```python
from build123d import *

# Parameters (mm, degrees)
F1_DEPTH = 101.6
F2_W     = 62.789462
F2_H     = 290.428608
F3_DEPTH = 76.2
F4_R     = 26.772602
F5_DEPTH = 101.6
F6_R     = 12.094446
F6_R_2   = 13.485849
F7_DEPTH = 101.6


with BuildPart() as f1:
    # F0 (on Front) → F1 (new body)
    with BuildSketch(Plane.XZ):
        with BuildLine():
            Line((27.304832, -72.607152), (27.304832, 72.607152))
            ThreePointArc((27.304832, 72.607152), (0, 99.911984), (-27.304832, 72.607152))
            Line((-27.304832, 72.607152), (-27.304832, -72.607152))
            ThreePointArc((-27.304832, -72.607152), (0, -99.911984), (27.304832, -72.607152))
        make_face()
    extrude(amount=-F1_DEPTH)

    # F2 (on face) → F3 (cut)
    with BuildSketch(Plane.YZ.offset(27.304832)):
        with Locations((50.8, 72.607152)):
            Rectangle(F2_W, F2_H)
    extrude(amount=-F3_DEPTH, mode=Mode.SUBTRACT)

    # F4 (on Front) → F5 (join)
    with BuildSketch(Plane.XZ):
        with Locations((0, -72.568707)):
            Circle(F4_R)
    extrude(amount=-F5_DEPTH)

    # F6 (on face) → F7 (cut)
    with BuildSketch(Plane.XZ):
        with Locations((0, 75.886309)):
            Circle(F6_R)
        with Locations((0, -72.607152)):
            Circle(F6_R_2)
    extrude(amount=-F7_DEPTH, mode=Mode.SUBTRACT)


solid = f1.part
```
CAD build for the part. Positions are in the model's coordinates, mm. Coordinates: 2 decimals unless noted, no trailing zeros. Write each loop counter-clockwise with the first axis right and the second up, starting at its lowest first coordinate (ties: lowest second). Pieces come first, ordered by that corner, then holes.
(1) Flat gauge pins, fed straight in: pin 1 (1.5 mm diameter, centred on y = 79.5, z = -56, fed in from -X); pin 2 (8 mm diameter, centred on y = 36, z = -46.5, fed in from -X); pin 3 (2 mm diameter, centred on x = 2.5, y = 74, fed in from +Z). Where does each tip first touch, or does it go through?
(2) Cut at B-B, the plane z = 26. List the corners of the cut face in (x, y), and give its area (3 significant figures).
(3) Cut at D-D, the plane y = 13. List the corners of the cut face in (x, z).
(4) Cut at A-A, the plane x = 0. List the corners of the cut face in (y, z).
(5) Two-plate mould, pull along Y, no slides. Class faces 1 (the face through (0, 0, 1)), 2 (the face through (0, 82.195, 12)), 3 (the face through (-0.6, 50.089, -99.905)): +Y half, -Y half, draft (parallel to the pull), parting line (faces both ways), or undercut.
(6) Cut at C-C, the plane y = 62.5. List the corners of the cut face in (x, z), and give its area (3 significant figures).
(7) Drill centre lines: probe 1 along Z at (x, y) = (0, 93); probe 2 along Z at (x, y) = (0, 47); probe 3 along Y at (x, z) = (-18, 41). Where is each one in solid material? Low to high.
Geometry says:
1. pin 1: stops at x = -21.6
1. pin 2: stops at x = -15.16
1. pin 3: stops at z = -45.84
2. outline: (-27.3, 0) - (27.3, 0) - (27.3, 19.41) - (-27.3, 19.41) - close; (-27.3, 82.19) - (27.3, 82.19) - (27.3, 101.6) - (-27.3, 101.6) - close
2. area: 2,120 mm2
3. outline: (-27.3, -72.61) arc R27.3 ccw to (27.3, -72.61) - (27.3, 72.61) arc R27.3 ccw to (-27.3, 72.61) - close; hole circle Ø26.97 at (0, -72.61); hole circle Ø24.19 at (0, 75.89)
4. outline: (0, -99.91) - (101.6, -99.91) - (101.6, -86.09) - (0, -86.09) - close; (0, -59.12) - (101.6, -59.12) - (101.6, 63.79) - (82.19, 63.79) - (82.19, -45.8) - (19.41, -45.8) - (19.41, 63.79) - (0, 63.79) - close; (0, 87.98) - (19.41, 87.98) - (19.41, 99.91) - (0, 99.91) - close; (82.19, 87.98) - (101.6, 87.98) - (101.6, 99.91) - (82.19, 99.91) - close
5. face 1: -Y half
5. face 2: undercut
5. face 3: draft
6. outline: (-27.3, -72.61) arc R27.3 ccw to (27.3, -72.61) - (26.77, -72.61) arc R26.77 ccw to (-26.77, -72.61) - close; hole circle Ø26.97 at (0, -72.61)
6. area: 1,730 mm2
7. probe 1: z = -99.91 to -86.09, -59.12 to 63.79, 87.98 to 99.91
7. probe 2: z = -99.91 to -86.09, -59.12 to -45.8
7. probe 3: y = 0 to 19.41, 82.19 to 101.6
